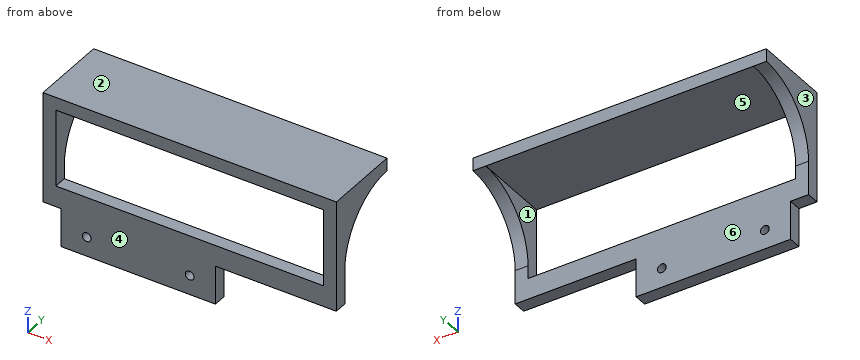
from build123d import *

# Parameters (mm, degrees)
SKETCH1_W           = 104
SKETCH1_H           = 30
SKETCH1_R           = 1.7
BOSS_EXTRUDE1_DEPTH = 5
BOSS_EXTRUDE2_DEPTH = 25
FILLET1_R           = 25


with BuildPart() as part:
    # Sketch1 → Boss-Extrude1 (new body)
    with BuildSketch(Plane(origin=(0, 0, 0), x_dir=(1, 0, 0), z_dir=(0, 1, 0))):
        Polygon((67, -8.528010066), (7, -8.528010066), (7, -23.528010066), (0, -23.528010066), (0, -66.703010066), (114, -66.703010066), (114, -23.528010066), (67, -23.528010066), align=None)
        with Locations((57, -46.703010066)):
            Rectangle(SKETCH1_W, SKETCH1_H, mode=Mode.SUBTRACT)
        with Locations(Location((17, -16.028010066, 0), (0, 0, 270))):
            Circle(SKETCH1_R, mode=Mode.SUBTRACT)
        with Locations(Location((57, -16.028010066, 0), (0, 0, 270))):
            Circle(SKETCH1_R, mode=Mode.SUBTRACT)
    extrude(amount=BOSS_EXTRUDE1_DEPTH)

    # Sketch2 → Boss-Extrude2 (add)
    with BuildSketch(Plane(origin=(0, 5, 0), x_dir=(1, 0, 0), z_dir=(0, 1, 0))):
        Polygon((5, -61.703010066), (0, -61.703010066), (0, -66.703010066), (114, -66.703010066), (114, -61.703010066), align=None)
    extrude(amount=BOSS_EXTRUDE2_DEPTH)

    # Fillet1
    fillet1_edges = [part.edges().sort_by_distance(p)[0] for p in [
        (2.5, 5, 61.703010066),
        (111.5, 5, 61.703010066),
    ]]
    fillet(fillet1_edges, radius=FILLET1_R - 0.0001)  # a hair under: the kernel refuses the full size


solid = part.part
Part model, mm, in its own coordinate system. Face numbers are marked on the shaded views. A direction names the side the tool comes from. Round coordinates to 2 decimals unless told otherwise and drop trailing zeros. Write each loop counter-clockwise with the first axis right and the second up, starting at its lowest first coordinate (ties: lowest second). Pieces come first, ordered by that corner, then holes. Notation, with made-up numbers: M 19,-34 L 57,-34 A35 cw 57,4 Z; hole C 85.25,-37 d2. An arc over 180 degrees is marked long. Return JSON: item names as keys, results as strings. Group by question number.
(1) Saw through at A-A on x = 78.5. Write the cut outline in (y, z).
(2) Saw through at C-C on y = 2.75. Write the cut outline in (x, z).
(3) Pin check, flat tips, straight feed: pin 1 Ø10 at (x, y) = (22.5, 17.5) entering from -Z; pin 2 Ø1.5 at (x, y) = (5, 2.5) entering from -Z; pin 3 Ø8 at (x, z) = (99.5, 39) entering from -Y; pin 4 Ø1.5 at (y, z) = (3.5, 19) entering from -X. Stop position of each tip, or through.
(4) Which spindle directions (+Z, -Z, +X, -X, +Y, -Y) get a long thin tool onto all of the face, cutting with end or side? Do the marked faces 4, 5 and 6. Say none if no direction does.
(5) Saw through at B-B on x = 57. Write the cut outline in (y, z), then the cut area to 3 significant figures.
(6) Saw through at D-D on z = 38.5. Write the cut outline in (x, y).
(7) Drill centre lines: probe 1 along Z at (x, y) = (66, 3.5); probe 2 along Z at (x, y) = (68.5, 4); probe 3 along X at (y, z) = (11.25, 59). Where is each one in solid material? Low to high.
(8) Two-plate mould, pull along Z, no slides. Class the marked faces 1, 2 and 3: +Z half, -Z half, draft (parallel to the pull), parting line (faces both ways), or undercut.
Returned:
{
 "1": {"outline": "M 0,23.53 L 5,23.53 L 5,31.7 L 0,31.7 Z; M 0,61.7 L 30,61.7 L 30,66.7 L 0,66.7 Z"},
 "2": {"outline": "M 0,23.53 L 7,23.53 L 7,8.53 L 67,8.53 L 67,23.53 L 114,23.53 L 114,66.7 L 0,66.7 Z; hole M 5,31.7 L 109,31.7 L 109,61.7 L 5,61.7 Z; hole C 17,16.03 d3.4; hole C 57,16.03 d3.4"},
 "3": {"pin 1": "z = 61.7", "pin 2": "z = 23.53", "pin 3": "through", "pin 4": "x = 7"},
 "4": {"face 4": "+Z, -Z, +X, -X, -Y", "face 5": "+Y, -Y", "face 6": "-Z, +X, -X, +Y"},
 "5": {"outline": "M 0,8.53 L 5,8.53 L 5,14.33 L 0,14.33 Z; M 0,17.73 L 5,17.73 L 5,31.7 L 0,31.7 Z; M 0,61.7 L 30,61.7 L 30,66.7 L 0,66.7 Z", "area": "249 mm²"},
 "6": {"outline": "M 0,0 L 5,0 L 5,5.06 L 0,5.06 Z; M 109,0 L 114,0 L 114,5.06 L 109,5.06 Z"},
 "7": {"probe 1": "8.53 to 31.7, 61.7 to 66.7", "probe 2": "23.53 to 31.7, 61.7 to 66.7", "probe 3": "0 to 5, 109 to 114"},
 "8": {"face 1": "undercut", "face 2": "+Z half", "face 3": "draft"}
}
